```python
from build123d import *

# Parameters (mm, degrees)
SKETCH1_W       = 36.8
SKETCH1_H       = 22.4
EXTRUDE1_DEPTH  = 9.3
FILLET1_R       = 5
SKETCH2_R       = 1.35
EXTRUDE2_DEPTH  = 1.55
SKETCH3_R       = 3.65
SKETCH3_R_2     = 2.5
EXTRUDE3_DEPTH  = 0.3
SKETCH4_R       = 1
EXTRUDE4_DEPTH  = 8.7
SKETCH6_R       = 2
EXTRUDE5_DEPTH  = 1
SKETCH7_R       = 1.5
EXTRUDE6_DEPTH  = 19.6
SKETCH8_R       = 2
EXTRUDE7_DEPTH  = 0.5
EXTRUDE8_DEPTH  = 0.5
SKETCH10_R      = 0.75
EXTRUDE9_DEPTH  = 0.5
EXTRUDE11_DEPTH = 12.1
EXTRUDE12_DEPTH = 15
SKETCH14_R      = 4
EXTRUDE13_DEPTH = 1
SKETCH15_R      = 1
EXTRUDE14_DEPTH = 1
SKETCH16_W      = 2
SKETCH16_H      = 0.5
EXTRUDE15_DEPTH = 3
SKETCH17_W      = 1
SKETCH17_H      = 2
EXTRUDE16_DEPTH = 18.618894796


with BuildPart() as part:
    # Sketch1 → Extrude1 (new body, symmetric)
    with BuildSketch(Plane(origin=(0, 0, 0), x_dir=(1, 0, 0), z_dir=(0, 1, 0))):
        with Locations((18.4, 11.2)):
            Rectangle(SKETCH1_W, SKETCH1_H)
    extrude(amount=EXTRUDE1_DEPTH, both=True)

    # Fillet1
    fillet1_edges = [part.edges().sort_by_distance(p)[0] for p in [
        (36.8, 0, -22.4),
        (36.8, 0, 0),
    ]]
    fillet(fillet1_edges, radius=FILLET1_R)

    # Sketch2 → Extrude2 (add, symmetric)
    with BuildSketch(Plane(origin=(0, 0, 0), x_dir=(1, 0, 0), z_dir=(0, 1, 0))):
        with BuildLine():
            Line((36.8, 14.2), (40.004789912, 13.495144254))
            ThreePointArc((40.004789912, 13.495144254), (41.85, 11.2), (40.004789912, 8.904855746))
            Line((40.004789912, 8.904855746), (36.8, 8.2))
            Line((36.8, 8.2), (36.8, 14.2))
        make_face()
        with Locations(Location((39.5, 11.2, 0), (0, 0, 270))):  # turned: the seam where the file's is
            Circle(SKETCH2_R, mode=Mode.SUBTRACT)
    extrude(amount=EXTRUDE2_DEPTH, both=True)

    # Sketch3 → Extrude3 (add)
    with BuildSketch(Plane(origin=(0, 9.3, 0), x_dir=(1, 0, 0), z_dir=(0, 1, 0))):
        with Locations(Location((25.45, 11.2, 0), (0, 0, 90))):  # turned: the seam where the file's is
            Circle(SKETCH3_R)
        with Locations(Location((13.1, 11.2, 0), (0, 0, 90))):  # turned: the seam where the file's is
            Circle(SKETCH3_R_2)
    extrude(amount=EXTRUDE3_DEPTH)

    # Sketch4 → Extrude4 (add)
    with BuildSketch(Plane(origin=(0, 9.6, 0), x_dir=(1, 0, 0), z_dir=(0, 1, 0))):
        with BuildLine():
            Line((23.062532723, 8.85), (27.837467277, 8.85))
            ThreePointArc((27.837467277, 8.85), (28.8, 11.2), (27.837467277, 13.55))
            Line((27.837467277, 13.55), (23.062532723, 13.55))
            ThreePointArc((23.062532723, 13.55), (22.1, 11.2), (23.062532723, 8.85))
        make_face()
        with Locations(Location((25.45, 11.2, 0), (0, 0, 270))):  # turned: the seam where the file's is
            Circle(SKETCH4_R, mode=Mode.SUBTRACT)
    extrude(amount=EXTRUDE4_DEPTH)

    # Sketch6 → Extrude5 (add)
    with BuildSketch(Plane(origin=(0, 9.6, 0), x_dir=(1, 0, 0), z_dir=(0, 1, 0))):
        with Locations(Location((13.1, 11.2, 0), (0, 0, 270))):  # turned: the seam where the file's is
            Circle(SKETCH6_R)
    extrude(amount=EXTRUDE5_DEPTH)

    # Sketch7 → Extrude6 (cut, through all)
    with BuildSketch(Plane(origin=(0, 9.3, 0), x_dir=(1, 0, 0), z_dir=(0, 1, 0))):
        with Locations(Location((4, 20.4, 0), (0, 0, 270))):  # turned: the seam where the file's is
            Circle(SKETCH7_R)
        with Locations(Location((4, 2, 0), (0, 0, 270))):  # turned: the seam where the file's is
            Circle(SKETCH7_R)
    extrude(amount=-EXTRUDE6_DEPTH, mode=Mode.SUBTRACT)

    # Sketch8 → Extrude7 (cut)
    with BuildSketch(Plane(origin=(0, 9.3, 0), x_dir=(1, 0, 0), z_dir=(0, 1, 0))):
        with Locations(Location((2.5, 16.9, 0), (0, 0, 270))):  # turned: the seam where the file's is
            Circle(SKETCH8_R)
        with Locations(Location((2.5, 5.5, 0), (0, 0, 270))):  # turned: the seam where the file's is
            Circle(SKETCH8_R)
    extrude(amount=-EXTRUDE7_DEPTH, mode=Mode.SUBTRACT)

    # Sketch9 → Extrude8 (cut)
    with BuildSketch(Plane(origin=(0, 8.8, 0), x_dir=(1, 0, 0), z_dir=(0, 1, 0))):
        with BuildLine():
            Line((2, 7.019868415), (2, 6))
            Line((2, 6), (0.980131585, 6))
            ThreePointArc((0.980131585, 6), (0.9, 5.5), (0.980131585, 5))
            Line((0.980131585, 5), (2, 5))
            Line((2, 5), (2, 3.980131585))
            ThreePointArc((2, 3.980131585), (2.5, 3.9), (3, 3.980131585))
            Line((3, 3.980131585), (3, 5))
            Line((3, 5), (4.019868415, 5))
            ThreePointArc((4.019868415, 5), (4.1, 5.5), (4.019868415, 6))
            Line((4.019868415, 6), (3, 6))
            Line((3, 6), (3, 7.019868415))
            ThreePointArc((3, 7.019868415), (2.5, 7.1), (2, 7.019868415))
        make_face()
        with BuildLine():
            Line((4.019868415, 17.4), (3, 17.4))
            Line((3, 17.4), (3, 18.419868415))
            ThreePointArc((3, 18.419868415), (2.5, 18.5), (2, 18.419868415))
            Line((2, 18.419868415), (2, 17.4))
            Line((2, 17.4), (0.980131585, 17.4))
            ThreePointArc((0.980131585, 17.4), (0.9, 16.9), (0.980131585, 16.4))
            Line((0.980131585, 16.4), (2, 16.4))
            Line((2, 16.4), (2, 15.380131585))
            ThreePointArc((2, 15.380131585), (2.5, 15.3), (3, 15.380131585))
            Line((3, 15.380131585), (3, 16.4))
            Line((3, 16.4), (4.019868415, 16.4))
            ThreePointArc((4.019868415, 16.4), (4.1, 16.9), (4.019868415, 17.4))
        make_face()
    extrude(amount=-EXTRUDE8_DEPTH, mode=Mode.SUBTRACT)

    # Sketch10 → Extrude9 (add)
    with BuildSketch(Plane(origin=(0, 9.3, 0), x_dir=(1, 0, 0), z_dir=(0, 1, 0))):
        with Locations(Location((1.3, 21.1, 0), (0, 0, 90))):  # turned: the seam where the file's is
            Circle(SKETCH10_R)
        with Locations(Location((1.3, 1.3, 0), (0, 0, 90))):  # turned: the seam where the file's is
            Circle(SKETCH10_R)
    extrude(amount=EXTRUDE9_DEPTH)

    # Sketch12 → Extrude11 (add)
    with BuildSketch(Plane.ZY):
        with BuildLine():
            Line((-19.038367177, 8), (-3.361632823, 8))
            ThreePointArc((-3.361632823, 8), (0, 0), (-3.361632823, -8))
            Line((-3.361632823, -8), (-19.038367177, -8))
            ThreePointArc((-19.038367177, -8), (-22.4, 0), (-19.038367177, 8))
        make_face()
    extrude(amount=EXTRUDE11_DEPTH)

    # Sketch13 → Extrude12 (add)
    with BuildSketch(Plane.ZY.offset(12.1)):
        with BuildLine():
            Line((-18.618894796, -7), (-3.781105204, -7))
            ThreePointArc((-3.781105204, -7), (-1, 0), (-3.781105204, 7))
            Line((-3.781105204, 7), (-18.618894796, 7))
            ThreePointArc((-18.618894796, 7), (-21.4, 0), (-18.618894796, -7))
        make_face()
    extrude(amount=EXTRUDE12_DEPTH)

    # Sketch14 → Extrude13 (add)
    with BuildSketch(Plane.ZY.offset(27.1)):
        with Locations((-11.2, 0)):
            Circle(SKETCH14_R)
    extrude(amount=EXTRUDE13_DEPTH)

    # Sketch15 → Extrude14 (add)
    with BuildSketch(Plane.ZY.offset(28.1)):
        with Locations((-11.2, 0)):
            Circle(SKETCH15_R)
    extrude(amount=EXTRUDE14_DEPTH)

    # Sketch16 → Extrude15 (add)
    with BuildSketch(Plane(origin=(0, 7, 0), x_dir=(1, 0, 0), z_dir=(0, 1, 0))):
        with Locations((-25.6, 17.368894796)):
            Rectangle(SKETCH16_W, SKETCH16_H)
        with Locations((-25.6, 5.031105204)):
            Rectangle(SKETCH16_W, SKETCH16_H)
    extrude(amount=EXTRUDE15_DEPTH)

    # Sketch17 → Extrude16 (cut, through all)
    with BuildSketch(Plane.XY.offset(-4.781105204)):
        with Locations((-25.6, 8.5)):
            Rectangle(SKETCH17_W, SKETCH17_H)
    extrude(amount=-EXTRUDE16_DEPTH, mode=Mode.SUBTRACT)


solid = part.part
```
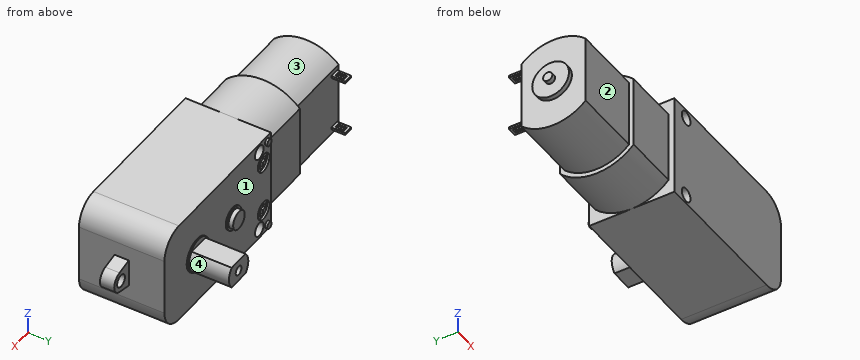
Work out the finished part from the listing and answer in its coordinate system (mm). Face numbers are marked on the shaded views. A direction names the side the tool comes from. Coordinates: 2 decimals unless noted, no trailing zeros. Loops run counter-clockwise (first coordinate to the right, second up) from the corner with the lowest first, then second, coordinate; pieces in that order, holes last. Notation, with made-up numbers: M 72,69.5 L 103,69.5 A10 cw 103,82.5 Z; hole C -20.5,-21 d2. An arc over 180 degrees is marked long. Use CSV: the item, a comma, the result in double quotes. Start each with the question number.
(1) Find section B-B, the plane y = 3. Give the vertices of the cut face in (x, z).
(2) Consider line 1 (X direction, y = 15.5, z = -11.2); line 2 (X direction, y = 0.25, z = -11.2); line 3 (Y direction, x = -1.5, z = -7.25). Determine where each line is inside the solid, lowest interval first.
(3) Find section D-D, the plane y = 6. Give the vertices of the cut face in (x, z), then the cut area to 3 significant figures.
(4) Find section A-A, the plane x = 13.1. Give the vertices of the cut face in (y, z), then the cut area to 3 significant figures.
(5) Given pin 1 Ø2 at (x, z) = (-4.5, -9.5) entering from +Y; pin 2 Ø2.5 at (y, z) = (1.5, -13) entering from -X; pin 3 Ø1 at (x, y) = (-26, 8) entering from -Z, each flat-ended and moving along its own axis, determine where each tip first touches the part or whether it passes through.
(6) Find section C-C, the plane y = 13. Give the vertices of the cut face in (x, z), then the cut area to 3 significant figures.
(7) For the marked faces 1, 2, 3 and 4, determine the directions among +Z, -Z, +X, -X, +Y, -Y from which every point of the face is accessible in a straight line to the end or side of a thin tool.
Recorded:
1,outline,"M -28.1,-13.85 L -27.1,-13.85 L -27.1,-20.95 L -12.1,-20.95 L -12.1,-21.99 L 0,-21.99 L 0,-22.4 L 31.8,-22.4 A5 ccw 36.8,-17.4 L 36.8,-5 A5 ccw 31.8,0 L 0,0 L 0,-0.41 L -12.1,-0.41 L -12.1,-1.45 L -27.1,-1.45 L -27.1,-8.55 L -28.1,-8.55 Z; hole C 4,-20.4 d3; hole C 4,-2 d3"
2,line 1,"x = 22.1 to 24.45, 26.45 to 28.8"
2,line 2,"x = -29.1 to 38.15, 40.85 to 41.85"
2,line 3,"y = -8 to 8"
3,outline,"M -27.1,-19.45 L -12.1,-19.45 L -12.1,-20.66 L 0,-20.66 L 0,-22.4 L 31.8,-22.4 A5 ccw 36.8,-17.4 L 36.8,-5 A5 ccw 31.8,0 L 0,0 L 0,-1.74 L -12.1,-1.74 L -12.1,-2.95 L -27.1,-2.95 Z; hole C 4,-20.4 d3; hole C 4,-2 d3"
3,area,"1,280 mm^2"
4,outline,"M -9.3,-22.4 L 9.3,-22.4 L 9.3,-13.7 L 9.6,-13.7 L 9.6,-13.2 L 10.6,-13.2 L 10.6,-9.2 L 9.6,-9.2 L 9.6,-8.7 L 9.3,-8.7 L 9.3,0 L -9.3,0 Z"
4,area,"422 mm^2"
5,pin 1,"stops at y = 8"
5,pin 2,"stops at x = -28.1"
5,pin 3,"stops at z = -17.62"
6,outline,"M 23.06,-13.55 L 27.84,-13.55 A3.35 ccw 27.84,-8.85 L 23.06,-8.85 A3.35 ccw Z; hole C 25.45,-11.2 d2"
6,area,"25.5 mm^2"
7,face 1,"+Y"
7,face 2,"+Z, -Z, -X, -Y"
7,face 3,"+Z, -X"
7,face 4,"+X, +Y"
